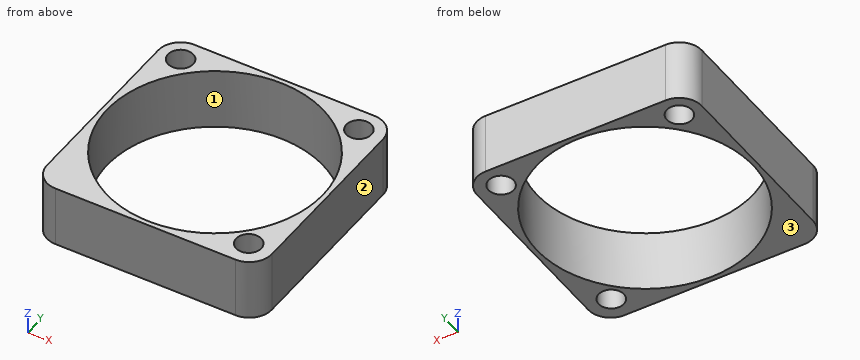
```python
from build123d import *

# Parameters (mm, degrees)
SKETCH1_W           = 25
SKETCH1_H           = 25
BOSS_EXTRUDE1_DEPTH = 6.8325
SKETCH2_R           = 12
CUT_EXTRUDE1_DEPTH  = 7.8325
SKETCH3_R           = 1.4
CUT_EXTRUDE2_DEPTH  = 7.8325
FILLET1_R           = 2.5


with BuildPart() as part:
    # Sketch1 → Boss-Extrude1 (new body)
    with BuildSketch(Plane.XY):
        with Locations((12.5, 12.5)):
            Rectangle(SKETCH1_W, SKETCH1_H)
    extrude(amount=BOSS_EXTRUDE1_DEPTH)

    # Sketch2 → Cut-Extrude1 (cut, through all)
    with BuildSketch(Plane.XY.offset(6.8325)):
        with Locations((12.5, 12.5)):
            Circle(SKETCH2_R)
    extrude(amount=-CUT_EXTRUDE1_DEPTH, mode=Mode.SUBTRACT)

    # Sketch3 → Cut-Extrude2 (cut, through all)
    with BuildSketch(Plane.XY.offset(6.8325)):
        with Locations((2.5, 22.5)):
            Circle(SKETCH3_R)
        with Locations((22.312, 22.5)):
            Circle(SKETCH3_R)
        with Locations((22.312, 2.688)):
            Circle(SKETCH3_R)
    extrude(amount=-CUT_EXTRUDE2_DEPTH, mode=Mode.SUBTRACT)

    # Fillet1
    fillet1_edges = [part.edges().sort_by_distance(p)[0] for p in [
        (0, 25, 3.41625),
        (25, 25, 3.41625),
        (25, 0, 3.41625),
        (0, 0, 3.41625),
    ]]
    fillet(fillet1_edges, radius=FILLET1_R)


solid = part.part
```
The model under review builds one solid part; all positions refer to its coordinate system, in mm. Face numbers are marked on the shaded views. Round coordinates to 2 decimals unless told otherwise and drop trailing zeros. Write each loop counter-clockwise with the first axis right and the second up, starting at its lowest first coordinate (ties: lowest second). Pieces come first, ordered by that corner, then holes. Notation, with made-up numbers: (-6.5, -20) - (5.5, -20) arc R27 ccw to (5.5, 11) - close; hole circle Ø9 at (39.25, 11.25). An arc over 180 degrees is marked (long way). Use one line per item in the form item = value.
Q1. Consider section A-A (x = 12.5). State the section outline as (y, z) points.
Answer key:
outline = (0, 0) - (0.5, 0) - (0.5, 6.83) - (0, 6.83) - close; (24.5, 0) - (25, 0) - (25, 6.83) - (24.5, 6.83) - close
Q2. For line 1 (Y direction, x = 22, z = 6); line 2 (X direction, y = 22.25, z = 6); line 3 (Y direction, x = 12.5, z = 5), list the stretches that pass through material, from the lowest coordinate up. Write a range as [from, to].
Answer key:
line_1 = [0, 1.32], [4.05, 5.17], [19.83, 21.14], [23.86, 25]
line_2 = [0, 1.12], [3.88, 5.5], [19.5, 20.93], [23.69, 25]
line_3 = [0, 0.5], [24.5, 25]
Q3. Consider section B-B (y = 3.25). State the section outline as (x, z) points.
Answer key:
outline = (0, 0) - (4.86, 0) - (4.86, 6.83) - (0, 6.83) - close; (20.14, 0) - (21.03, 0) - (21.03, 6.83) - (20.14, 6.83) - close; (23.59, 0) - (25, 0) - (25, 6.83) - (23.59, 6.83) - close
Q4. Consider section C-C (x = 2). State the section outline as (y, z) points.
Answer key:
outline = (0.05, 0) - (6.69, 0) - (6.69, 6.83) - (0.05, 6.83) - close; (18.31, 0) - (21.19, 0) - (21.19, 6.83) - (18.31, 6.83) - close; (23.81, 0) - (24.95, 0) - (24.95, 6.83) - (23.81, 6.83) - close
Q5. Draft analysis for pull direction X (two halves, no side actions). For the marked faces 1, 2 and 3, state which applies: +X half, -X half, draft (parallel to the pull), parting line (faces both ways), or undercut.
Answer key:
face_1 = undercut
face_2 = +X half
face_3 = draft
Q6. Consider section D-D (y = 20.25). State the section outline as (x, z) points.
Answer key:
outline = (0, 0) - (3.34, 0) - (3.34, 6.83) - (0, 6.83) - close; (21.66, 0) - (25, 0) - (25, 6.83) - (21.66, 6.83) - close
